The listing builds one solid part. Answer for the finished solid, in the listing's coordinates (mm). A direction names the side the tool comes from. Coordinates: 2 decimals unless noted, no trailing zeros. Order: outer loops, then holes, each group sorted by start corner. A loop starts at its lowest first (then second) coordinate and runs counter-clockwise, first axis right, second up. Notation, with made-up numbers: (14.5, 55) -> (65.5, 55) arc R24 cw to (65.5, 73) -> close; hole circle Ø6 at (-1, 0). An arc over 180 degrees is marked (long way). Write each question's results on one line, items separated by ' | '. Start each with the question number.
(1) A tool of negligible diameter and unlimited length cuts with its end or side. For faces 5 (the face through (9, 0, 2.54)), 6 (the face through (1.664, -6, 1)), 7 (the face through (-1.664, 3.1, 5.6)), 8 (the face through (11, -10.102, 1)), 9 (the face through (0, -1, 0)), from which of +Z, -Z, +X, -X, +Y, -Y can it reach the whole face along a straight path? Write none if from no direction.
(2) Given pin 1 (3 mm diameter, centred on x = -13.5, y = 7, fed in from -Z); pin 2 (0.9 mm diameter, centred on x = 6.5, z = -1, fed in from -Y); pin 3 (4 mm diameter, centred on y = 0.5, z = 7.5, fed in from +X), each flat-ended and moving along its own axis, determine where each tip first touches the part or whether it passes through.
(3) Straight lines are drawn through the part: L1, parallel to Y at x = 11, z = 0.75; L2, parallel to X at y = -3.25, z = 2.5; L3, parallel to X at y = -6.5, z = 1.25. For each, find the intervals that lie inside material, in ascending order.
(4) The part is cut by section B-B, the plane y = -6.5. Give the vertices of the cut face in (x, z), then the cut area to 3 significant figures.
(5) Determine the mould class of faces 1 (the face through (0, 10.102, -1)), 2 (the face through (9.5, -2.53, 1.25)), 3 (the face through (1.664, 3.1, 5.6)), 4 (the face through (-12.5, -2.53, 1.25)) for opening direction Y: +Y half, -Y half, draft (parallel to the pull), parting line (faces both ways), or undercut.
(6) The part is cut by section C-C, the plane z = 6.75. Give the vertices of the cut face in (x, y).
(7) The part is cut by section D-D, the plane y = 5.5. Give the vertices of the cut face in (x, z), then the cut area to 3 significant figures.
(8) The part is cut by section A-A, the plane x = -11. Give the vertices of the cut face in (y, z).
```python
from build123d import *

# Parameters (mm, degrees)
SKETCH1_R           = 1.5
BOSS_EXTRUDE1_DEPTH = 2.54
SKETCH2_W           = 3.3274
SKETCH2_H           = 13.8539982
BOSS_EXTRUDE2_DEPTH = 7.9375
SKETCH3_R           = 1.5
CUT_EXTRUDE1_DEPTH  = 20.0137
FILLET1_R           = 2.54
FILLET3_R           = 2.54
BOSS_EXTRUDE3_DEPTH = 34.7


with BuildPart() as part:
    # Sketch1 → Boss-Extrude1 (new body)
    with BuildSketch(Plane.XY):
        Polygon((17.35, 10.1019991), (-17.35, 10.1019991), (-17.35, -10.1019991), (-1.6637, -10.1019991), (-1.6637, -3.7519991), (1.6637, -3.7519991), (1.6637, -10.1019991), (17.35, -10.1019991), align=None)
        with Locations((-11, -2.5980009)):
            Circle(SKETCH1_R, mode=Mode.SUBTRACT)
        with Locations((11, -2.5980009)):
            Circle(SKETCH1_R, mode=Mode.SUBTRACT)
    extrude(amount=BOSS_EXTRUDE1_DEPTH)

    # Sketch2 → Boss-Extrude2 (add)
    with BuildSketch(Plane.XY.offset(2.54)):
        with Locations((0, 3.175)):
            Rectangle(SKETCH2_W, SKETCH2_H)
    extrude(amount=BOSS_EXTRUDE2_DEPTH)

    # Sketch3 → Cut-Extrude1 (cut, through all)
    with BuildSketch(Plane.ZY.offset(1.6637)):
        with Locations((7.3025, 3.175)):
            Circle(SKETCH3_R)
    extrude(amount=-CUT_EXTRUDE1_DEPTH, mode=Mode.SUBTRACT)

    # Fillet1
    fillet1_edges = [part.edges().sort_by_distance(p)[0] for p in [
        (0, -3.7519991, 10.4775),
    ]]
    fillet(fillet1_edges, radius=FILLET1_R)

    # Fillet3
    fillet3_edges = [part.edges().sort_by_distance(p)[0] for p in [
        (-1.6637, -10.1019991, 1.27),
        (1.6637, -10.1019991, 1.27),
    ]]
    fillet(fillet3_edges, radius=FILLET3_R)

    # Sketch4 → Boss-Extrude3 (add)
    with BuildSketch(Plane(origin=(17.35, 0, 0), x_dir=(0, 0, -1), z_dir=(1, 0, 0))):
        Polygon((2.625150229, -12.101561201), (2.667, -10.1019991), (4.666562101, -10.143848871), (4.62471233, -12.143410972), align=None)
        Polygon((5.090296931, 10.1019991), (0, 10.1019991), (0, 8.1019991), (3.048, 8.1019991), (2.667, -10.1019991), (4.666562101, -10.143848871), align=None)
    extrude(amount=-BOSS_EXTRUDE3_DEPTH)


solid = part.part
```
Established:
1) face 5: +Z, +X, +Y, -Y | face 6: +Z, -Y | face 7: +Z, -X, +Y, -Y | face 8: +Z, +X, -X, -Y | face 9: +X, -X, -Y
2) pin 1: stops at z = -5.06 | pin 2: stops at y = 8.1 | pin 3: stops at x = 1.66
3) L1: y = -10.1 to -4.1, -1.1 to 10.1 | L2: x = -17.35 to -12.35, -9.65 to 9.65, 12.35 to 17.35 | L3: x = -17.35 to -1.66, 1.66 to 17.35
4) outline: (-17.35, -4.74) -> (17.35, -4.74) -> (17.35, -2.74) -> (-17.35, -2.74) -> close; (-17.35, 0) -> (-1.66, 0) -> (-1.66, 2.54) -> (-17.35, 2.54) -> close; (1.66, 0) -> (17.35, 0) -> (17.35, 2.54) -> (1.66, 2.54) -> close | area: 149 mm^2
5) face 1: +Y half | face 2: undercut | face 3: draft | face 4: undercut
6) outline: (-1.66, -3.75) -> (1.66, -3.75) -> (1.66, 1.78) -> (-1.66, 1.78) -> close; (-1.66, 4.57) -> (1.66, 4.57) -> (1.66, 10.1) -> (-1.66, 10.1) -> close
7) outline: (-17.35, -4.99) -> (17.35, -4.99) -> (17.35, -2.99) -> (-17.35, -2.99) -> close; (-17.35, 0) -> (17.35, 0) -> (17.35, 2.54) -> (1.66, 2.54) -> (1.66, 10.48) -> (-1.66, 10.48) -> (-1.66, 2.54) -> (-17.35, 2.54) -> close | area: 184 mm^2
8) outline: (-12.14, -4.62) -> (10.1, -5.09) -> (10.1, 2.54) -> (-1.1, 2.54) -> (-1.1, 0) -> (8.1, 0) -> (8.1, -3.05) -> (-12.1, -2.63) -> close; (-10.1, 0) -> (-4.1, 0) -> (-4.1, 2.54) -> (-10.1, 2.54) -> close
